```python
from build123d import *

# Parameters (mm, degrees)
SKIZZE1_W                       = 40
SKIZZE1_H                       = 125
SKIZZE1_R                       = 3.75
AUFSATZ_LINEAR_AUSTRAGEN1_DEPTH = 5
VERRUNDUNG1_R                   = 10


with BuildPart() as part:
    # Skizze1 → Aufsatz-Linear austragen1 (new body)
    with BuildSketch(Plane.XY):
        Rectangle(SKIZZE1_W, SKIZZE1_H)
        with Locations((0, 34)):
            Circle(SKIZZE1_R, mode=Mode.SUBTRACT)
        with Locations(Location((0, -34, 0), (0, 0, 180))):
            Circle(SKIZZE1_R, mode=Mode.SUBTRACT)
    extrude(amount=AUFSATZ_LINEAR_AUSTRAGEN1_DEPTH)

    # Verrundung1
    verrundung1_edges = [part.edges().sort_by_distance(p)[0] for p in [
        (-20, 62.5, 2.5),
        (20, 62.5, 2.5),
        (20, -62.5, 2.5),
        (-20, -62.5, 2.5),
    ]]
    fillet(verrundung1_edges, radius=VERRUNDUNG1_R)


solid = part.part
```
The listing builds one solid part. Answer for the finished solid, in the listing's coordinates (mm). Coordinates: 2 decimals unless noted, no trailing zeros. Loops run counter-clockwise (first coordinate to the right, second up) from the corner with the lowest first, then second, coordinate; pieces in that order, holes last. Notation, with made-up numbers: (16.5, 25) - (23.5, 25) arc R13 ccw to (23.5, 49) - close; hole circle Ø6 at (69, 83.25). An arc over 180 degrees is marked (long way). Use a Markdown table: item, result. Add a question column.
1) The mould has two halves that part along X. Classify faces 1 (the cylindrical face through (-17.15, -59.49, 2.54)), 2 (the cylindrical face through (0.81, -30.34, 2.46)), 3 (the flat face through (0, 62.5, 2)): released by +X, released by -X, zero draft, split by the parting line, or undercut.
2) The part is cut by section A-A, the plane x = 0. Give the vertices of the cut face in (y, z).
3) The part is cut by section B-B, the plane y = -34. Give the vertices of the cut face in (x, z).
4) Find the intervals of material crossed by line 1 (Y direction, x = 0, z = 2.8); line 2 (X direction, y = -34, z = 4.2); line 3 (Y direction, x = -1, z = 1.8), in increasing order.
5) The part is cut by section C-C, the plane z = 2.5. Give the vertices of the cut face in (x, y), and give its area (3 significant figures).
Here are the results:
| question | item | result |
|---|---|---|
| 1 | face 1 | released by -X |
| 1 | face 2 | undercut |
| 1 | face 3 | zero draft |
| 2 | outline | (-62.5, 0) - (-37.75, 0) - (-37.75, 5) - (-62.5, 5) - close; (-30.25, 0) - (30.25, 0) - (30.25, 5) - (-30.25, 5) - close; (37.75, 0) - (62.5, 0) - (62.5, 5) - (37.75, 5) - close |
| 3 | outline | (-20, 0) - (-3.75, 0) - (-3.75, 5) - (-20, 5) - close; (3.75, 0) - (20, 0) - (20, 5) - (3.75, 5) - close |
| 4 | line 1 | y = -62.5 to -37.75, -30.25 to 30.25, 37.75 to 62.5 |
| 4 | line 2 | x = -20 to -3.75, 3.75 to 20 |
| 4 | line 3 | y = -62.5 to -37.61, -30.39 to 30.39, 37.61 to 62.5 |
| 5 | outline | (-20, -52.5) arc R10 ccw to (-10, -62.5) - (10, -62.5) arc R10 ccw to (20, -52.5) - (20, 52.5) arc R10 ccw to (10, 62.5) - (-10, 62.5) arc R10 ccw to (-20, 52.5) - close; hole circle Ø7.5 at (0, -34); hole circle Ø7.5 at (0, 34) |
| 5 | area | 4,830 mm^2 |
